```python
from build123d import *

# Parameters (mm, degrees)
F0_R          = 5.3975
F1_DEPTH      = 6.35
F2_W          = 15.4239367694
F2_H          = 3.302921541
F3_DEPTH      = 25.4
F3_DEPTH_BACK = 25.4


with BuildPart() as f1:
    # F0 (on Top) → F1 (new body)
    with BuildSketch(Plane.XY):
        with BuildLine():
            Line((0, 9.525), (-12.6440079791, 9.525))
            Line((-12.6440079791, 9.525), (-12.6440079791, -9.525))
            Line((-12.6440079791, -9.525), (0, -9.525))
            ThreePointArc((0, -9.525), (9.525, 0), (0, 9.525))
        make_face()
        Circle(F0_R, mode=Mode.SUBTRACT)
        with BuildLine():
            Line((-12.6440079791, -9.525), (-12.6440079791, 9.525))
            ThreePointArc((-12.6440079791, 9.525), (-22.1690079791, 0), (-12.6440079791, -9.525))
        make_face()
    extrude(amount=F1_DEPTH)

    # F2 (on Front) → F3 (cut, two sides)
    with BuildSketch(Plane.XZ) as f3_sk:
        with Locations((-7.7119683847, 1.6514607705)):
            Rectangle(F2_W, F2_H)
    extrude(amount=-F3_DEPTH, mode=Mode.SUBTRACT)
    extrude(f3_sk.sketch, amount=F3_DEPTH_BACK, mode=Mode.SUBTRACT)


solid = f1.part
```
For this review, take the finished solid that the model builds, in its own axes (mm). A direction names the side the tool comes from. Coordinates: 2 decimals unless noted, no trailing zeros. Loops run counter-clockwise (first coordinate to the right, second up) from the corner with the lowest first, then second, coordinate; pieces in that order, holes last. Notation, with made-up numbers: (86, 73.5) - (131, 73.5) arc R19 cw to (131, 94.5) - close; hole circle Ø2 at (-33, 34.25). An arc over 180 degrees is marked (long way). Use one line per item in the form item = value. Start each with the question number.
1) For pin 1 (2.5 mm diameter, centred on y = -3.5, z = 2, fed in from +X); pin 2 (1 mm diameter, centred on x = -14, y = 3.5, fed in from -Z); pin 3 (1.5 mm diameter, centred on x = -17, z = 4, fed in from -Y); pin 4 (1.5 mm diameter, centred on x = -8.5, z = 2.5, fed in from +Y), all flat-tipped, find the tip position at first contact; note any pin that passes through.
2) To check wall thickness, follow probe 1 along Y at (x, z) = (0, 4.5) (1 decimal); probe 2 along X at (y, z) = (0, 4.5) (1 decimal); probe 3 along X at (y, z) = (0, 1.5) (1 decimal). State the ranges of each line that lie inside material, in increasing order. Write a range as from..to.
3) For faces 5 (the face through (6, 0, 0)), 6 (the face through (-15.424, 0, 2)), list the 3-axis set-ups (+Z, -Z, +X, -X, +Y, -Y) from which the entire face can be reached by the end or side of a thin tool; tool diameter is ignored.
4) Draft analysis for pull direction Y (two halves, no side actions). For faces 1 (the face through (-22.167, 0.209, 3.131)), 2 (the face through (5.15, 1.62, 3.84)), 3 (the face through (0, -7, 2)), 4 (the face through (-6, 9.525, 5)), state which applies: released by +Y, released by -Y, zero draft, split by the parting line, or undercut.
5) Take a section at C-C (x = -2). State the section outline as (y, z) points (3 decimals), plus the area to 3 significant figures.
From the geometry:
q1.pin_1 = 9.26
q1.pin_2 = 3.3
q1.pin_3 = -8.82
q1.pin_4 = through
q2.probe_1 = -9.5..-5.4, 5.4..9.5
q2.probe_2 = -22.2..-5.4, 5.4..9.5
q2.probe_3 = -22.2..-15.4, 5.4..9.5
q3.face_5 = -Z, +X, -X, +Y, -Y
q3.face_6 = -Z, +Y, -Y
q4.face_1 = split by the parting line
q4.face_2 = undercut
q4.face_3 = zero draft
q4.face_4 = released by +Y
q5.outline = (-9.525, 3.303) - (-5.013, 3.303) - (-5.013, 6.35) - (-9.525, 6.35) - close; (5.013, 3.303) - (9.525, 3.303) - (9.525, 6.35) - (5.013, 6.35) - close
q5.area = 27.5 mm2
